Job drawing, mm, ordinate dimensions from the low corner. One solid piece. A direction names the side the tool comes from. Give positions to 0.01 mm unless a question says otherwise; leave off trailing zeros. Order: outer loops, then holes, each group sorted by start corner. A loop starts at its lowest first (then second) coordinate and runs counter-clockwise, first axis right, second up. Notation, with made-up numbers: (80, 54.25) - (86, 54.25) arc R13 ccw to (86, 72.25) - close; hole circle Ø3 at (74, 40.5). An arc over 180 degrees is marked (long way). Use one line per item in the form item = value. Start each with the question number.
1. Drill centre lines: line 1 (Y direction, x = 23.5, z = 7); line 2 (X direction, y = 65.5, z = 13.5) (1 decimal); line 3 (Z direction, x = 94.5, y = 67.5). Where is each one in solid material? Low to high.
2. Band-saw the part on C-C, the plane z = 25.5. List the corners of the cut face in (x, y).
3. Band-saw the part on B-B, the plane x = 14. List the corners of the cut face in (y, z), plus the area to 3 significant figures.
4. Pin check, flat tips, straight feed: P1, Ø3, axis at y = 40.5, z = 8, coming from the -X side (1 decimal); P2, Ø12.5, axis at y = 54.5, z = 18, coming from the -X side; P3, Ø8, axis at x = 10, z = 16.5, coming from the +Y side. Stop position of each tip, or through.
5. Band-saw the part on A-A, the plane y = 54. List the corners of the cut face in (x, z), plus the area to 3 significant figures.
6. Band-saw the part on D-D, the plane y = 10.5. List the corners of the cut face in (x, z), plus the area to 3 significant figures.
7. Tool access for the marked faces 1, 2 and 3: list every direction of +Z, -Z, +X, -X, +Y, -Y with a clear straight run to the whole face (end or side of a thin tool).
8. Pull direction X, two halves, no side cores. Call the marked faces 4, 5, 6 and 7: +X half, -X half, draft (parallel to the pull), parting line (faces both ways), or undercut.
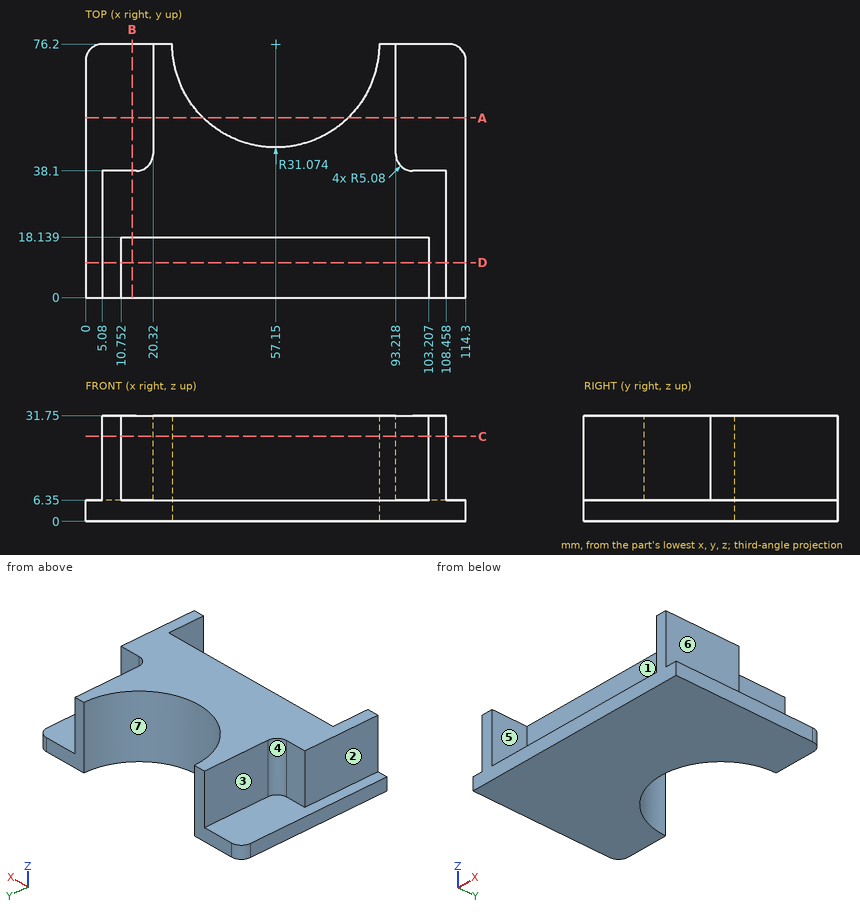
From the geometry:
q1.line_1 = 18.14 to 76.2
q1.line_2 = 20.3 to 28, 86.3 to 93.2
q1.line_3 = 0 to 6.35
q2.outline = (5.08, 0) - (10.75, 0) - (10.75, 18.14) - (103.21, 18.14) - (103.21, 0) - (108.46, 0) - (108.46, 38.1) - (98.3, 38.1) arc R5.08 cw to (93.22, 43.18) - (93.22, 76.2) - (88.22, 76.2) arc R31.07 cw to (26.08, 76.2) - (20.32, 76.2) - (20.32, 43.18) arc R5.08 cw to (15.24, 38.1) - (5.08, 38.1) - close
q3.outline = (0, 0) - (76.2, 0) - (76.2, 6.35) - (38.1, 6.35) - (38.1, 31.75) - (18.14, 31.75) - (18.14, 6.35) - (0, 6.35) - close
q3.area = 991 mm²
q4.P1 = 18.1
q4.P2 = 20.32
q4.P3 = 38.1
q5.outline = (0, 0) - (35.41, 0) - (35.41, 31.75) - (20.32, 31.75) - (20.32, 6.35) - (0, 6.35) - close; (78.89, 0) - (114.3, 0) - (114.3, 6.35) - (93.22, 6.35) - (93.22, 31.75) - (78.89, 31.75) - close
q5.area = 1,200 mm²
q6.outline = (0, 0) - (114.3, 0) - (114.3, 6.35) - (108.46, 6.35) - (108.46, 31.75) - (103.21, 31.75) - (103.21, 6.35) - (10.75, 6.35) - (10.75, 31.75) - (5.08, 31.75) - (5.08, 6.35) - (0, 6.35) - close
q6.area = 1,000 mm²
q7.face_1 = +Z, -Y
q7.face_2 = +Z, -X, +Y, -Y
q7.face_3 = +Z, -X, +Y
q8.face_4 = -X half
q8.face_5 = undercut
q8.face_6 = +X half
q8.face_7 = undercut
